from build123d import *

# Parameters (mm, degrees)
BOSS_EXTRUDE1_DEPTH = 450
SHELL1_T            = -0.35


with BuildPart() as part:
    # Sketch1 → Boss-Extrude1 (new body)
    with BuildSketch(Plane(origin=(0, 0, 0), x_dir=(1, 0, 0), z_dir=(0, 1, 0))):
        with BuildLine():
            Line((-350.175, 0), (-27.5, 0))
            ThreePointArc((-27.5, 0), (-19.445436483, 19.445436483), (0, 27.5))
            Line((0, 27.5), (0, 350.175))
            ThreePointArc((0, 350.175), (-247.611117102, 247.611117102), (-350.175, 0))
        make_face()
    extrude(amount=BOSS_EXTRUDE1_DEPTH)

    # Shell1
    shell1_openings = [part.faces().sort_by_distance(p)[0] for p in [
        (-113.973513396, 450, -113.973513396),
    ]]
    offset(amount=SHELL1_T, openings=shell1_openings, kind=Kind.INTERSECTION)


solid = part.part
Build history of the part. All positions in model axes, mm. A direction names the side the tool comes from. Give positions to 0.01 mm unless a question says otherwise; leave off trailing zeros. Order: outer loops, then holes, each group sorted by start corner. A loop starts at its lowest first (then second) coordinate and runs counter-clockwise, first axis right, second up. Notation, with made-up numbers: M 3.25,35 L 31.25,35 A20 ccw 31.25,64 Z; hole C 27.25,64.25 d2. An arc over 180 degrees is marked long. Put each result on its own line as item: value.
Item 1: 3-axis set-ups, long thin cutter, end or side, ignore diameter. For faces 4 (the flat face through (-191, 222, -0.35)), 5 (the cylindrical face through (-19.66, 221.85, -19.23)): which of +Z, -Z, +X, -X, +Y, -Y reach the whole face in a straight line?
From the geometry:
face 4: +Y
face 5: +Z, +X, +Y, -Y
Item 2: Probe line 1 (Y direction, x = -133, z = -168.5); line 2 (X direction, y = 20.5, z = -55); line 3 (Z direction, x = -295, y = 220.5). List the from-to ranges inside material, lowest first. Write a range as [from, to].
From the geometry:
line 1: y = [0, 0.35]
line 2: x = [-345.83, -345.47], [-0.35, 0]
line 3: z = [-188.67, -188.02], [-0.35, 0]
Item 3: Slice it at B-B, the plane z = -120. Write the cut outline in (x, y).
From the geometry:
outline: M -328.97,0 L 0,0 L 0,450 L -0.35,450 L -0.35,0.35 L -328.6,0.35 L -328.6,450 L -328.97,450 Z
Item 4: Slice it at C-C, the plane x = -89.5. Write the cut outline in (y, z).
From the geometry:
outline: M 0,-338.54 L 450,-338.54 L 450,-338.18 L 0.35,-338.18 L 0.35,-0.35 L 450,-0.35 L 450,0 L 0,0 Z
Item 5: Flat gauge pins, fed straight in: pin 1 Ø3 at (x, z) = (-101, -145) entering from +Y; pin 2 Ø1.5 at (y, z) = (317.5, -281.5) entering from -X; pin 3 Ø12 at (x, z) = (-277.5, -71) entering from -Y. Where does each tip first touch, or does it go through?
From the geometry:
pin 1: stops at y = 0.35
pin 2: stops at x = -209.29
pin 3: stops at y = 0
Item 6: Slice it at A-A, the plane y = 416. Write the cut outline in (x, z) (3 decimals).
From the geometry:
outline: M -350.175,0 A350.175 ccw 0,-350.175 L 0,-27.5 A27.5 cw -27.5,0 Z; hole M -349.825,-0.35 A349.825 ccw -0.35,-349.825 L -0.35,-27.848 A27.85 cw -27.848,-0.35 Z
Item 7: Two-plate mould, pull along X, no slides. Class faces 1 (the flat face through (0, 222, -187)), 2 (the flat face through (-139, 0, -139)), 3 (the cylindrical face through (-244.63, 222.03, -250.07)): +X half, -X half, draft (parallel to the pull), parting line (faces both ways), or undercut.
From the geometry:
face 1: +X half
face 2: draft
face 3: undercut
